```python
from build123d import *

# Parameters (mm, degrees)
SKETCH2_R           = 12.45
BOSS_EXTRUDE1_DEPTH = 16.915
SKETCH6_R           = 11
CUT_EXTRUDE2_DEPTH  = 15.5
BOSS_EXTRUDE2_START = 9
BOSS_EXTRUDE2_DEPTH = 9
SKETCH5_R           = 2.265
CUT_EXTRUDE1_DEPTH  = 33.574986186
CHAMFER1_SIZE       = 0.5
CHAMFER2_SIZE       = 0.5


with BuildPart() as part:
    # Sketch2 → Boss-Extrude1 (new body)
    with BuildSketch(Plane(origin=(0, 0, 0), x_dir=(1, 0, 0), z_dir=(0, 1, 0))):
        with Locations(Location((0, 0, 0), (0, 0, 270))):
            Circle(SKETCH2_R)
    extrude(amount=BOSS_EXTRUDE1_DEPTH)

    # Sketch6 → Cut-Extrude2 (cut)
    with BuildSketch(Plane.XZ):
        with Locations(Location((0, 0, 0), (0, 0, 270))):
            Circle(SKETCH6_R)
    extrude(amount=-CUT_EXTRUDE2_DEPTH, mode=Mode.SUBTRACT)

    # Sketch7 → Boss-Extrude2 (add)
    with BuildSketch(Plane.XZ.offset(-15.5).offset(BOSS_EXTRUDE2_START)):
        with BuildLine():
            Line((-4, 10.246950766), (-4, -10.246950766))
            ThreePointArc((-4, -10.246950766), (-11, 0), (-4, 10.246950766))
        make_face()
        with BuildLine():
            Line((4, 10.246950766), (4, -10.246950766))
            ThreePointArc((4, -10.246950766), (11, 0), (4, 10.246950766))
        make_face()
    extrude(amount=-BOSS_EXTRUDE2_DEPTH)

    # Sketch5 → Cut-Extrude1 (cut, through all)
    with BuildSketch(Plane(origin=(12.45, 0, 0), x_dir=(0, 0, -1), z_dir=(1, 0, 0))):
        with Locations((0, 9.95)):
            Circle(SKETCH5_R)
    extrude(amount=-CUT_EXTRUDE1_DEPTH, mode=Mode.SUBTRACT)

    # Chamfer1
    chamfer1_edges = [part.edges().sort_by_distance(p)[0] for p in [
        (0, 16.915, -12.45),
    ]]
    chamfer(chamfer1_edges, length=CHAMFER1_SIZE)

    # Chamfer2
    chamfer2_edges = [part.edges().sort_by_distance(p)[0] for p in [
        (0, 0, -12.45),
    ]]
    chamfer(chamfer2_edges, length=CHAMFER2_SIZE)


solid = part.part
```
The listing builds one solid part. Answer for the finished solid, in the listing's coordinates (mm). A direction names the side the tool comes from. Coordinates: 2 decimals unless noted, no trailing zeros. Write each loop counter-clockwise with the first axis right and the second up, starting at its lowest first coordinate (ties: lowest second). Pieces come first, ordered by that corner, then holes. Notation, with made-up numbers: (45.25, -11.75) - (57.25, -11.75) arc R32 cw to (57.25, 17.25) - close; hole circle Ø9 at (-10.5, 4). An arc over 180 degrees is marked (long way). Return JSON: item names as keys, results as strings. Group by question number.
1. Which of the six approach directions +Z, -Z, +X, -X, +Y, -Y give full straight-line access (tool end or side, diameter ignored) to faces 1 (the flat face through (7, 6.5, 0)), 2 (the cylindrical face through (-12.154, 8.346, -2.699))?
2. Straight lines are drawn through the part: L1, parallel to X at y = 15.25, z = 3.5; L2, parallel to Y at x = -7.75, z = 0 (3 decimals); L3, parallel to Y at x = -0.25, z = 8.25 (3 decimals). For each, find the intervals that lie inside material, in ascending order.
3. Given pin 1 (2.5 mm diameter, centred on x = 0, z = -4.5, fed in from -Y); pin 2 (7.5 mm diameter, centred on x = -6.5, z = 3, fed in from -Y); pin 3 (4 mm diameter, centred on y = 4, z = -2.5, fed in from +X), each flat-ended and moving along its own axis, determine where each tip first touches the part or whether it passes through.
4. A cutting plane is placed at D-D, the plane x = 0. Determine the outline of the cut face in (y, z) (3 decimals).
5. A cutting plane is placed at A-A, the plane z = 0. Determine the outline of the cut face in (x, y) (3 decimals), plus the area to 3 significant figures.
6. A cutting plane is placed at C-C, the plane y = 13. Determine the outline of the cut face in (x, z), plus the area to 3 significant figures.
7. A cutting plane is placed at B-B, the plane y = 9.95. Determine the outline of the cut face in (x, z) (3 decimals), plus the area to 3 significant figures.
8. Determine the mould class of faces 3 (the flat face through (0, 16.915, 0)), 4 (the flat face through (4, 13, 0)), 5 (the cylindrical face through (8.28, 7.74, 0.49)), 6 (the cylindrical face through (-8.17, 7.74, 0.49)) for opening direction Y: released by +Y, released by -Y, zero draft, split by the parting line, or undercut.
Ans:
{
 "1": {"face 1": "-Y", "face 2": "+Y, -Y"},
 "2": {"L1": "-11.95 to -4, 4 to 11.95", "L2": "6.5 to 7.685, 12.215 to 16.915", "L3": "15.5 to 16.915"},
 "3": {"pin 1": "y = 15.5", "pin 2": "y = 6.5", "pin 3": "x = 12.44"},
 "4": {"outline": "(0, -11.95) - (0.5, -12.45) - (16.415, -12.45) - (16.915, -11.95) - (16.915, 11.95) - (16.415, 12.45) - (0.5, 12.45) - (0, 11.95) - (0, 11) - (15.5, 11) - (15.5, -11) - (0, -11) - close"},
 "5": {"outline": "(-12.45, 0.5) - (-11.95, 0) - (-11, 0) - (-11, 6.5) - (-4, 6.5) - (-4, 7.685) - (-12.45, 7.685) - close; (-12.45, 12.215) - (-4, 12.215) - (-4, 15.5) - (4, 15.5) - (4, 12.215) - (12.45, 12.215) - (12.45, 16.415) - (11.95, 16.915) - (-11.95, 16.915) - (-12.45, 16.415) - close; (4, 6.5) - (11, 6.5) - (11, 0) - (11.95, 0) - (12.45, 0.5) - (12.45, 7.685) - (4, 7.685) - close", "area": "129 mm²"},
 "6": {"outline": "circle Ø24.9 at (0, 0); hole (-4, -10.25) arc R11 ccw to (4, -10.25) - (4, 10.25) arc R11 ccw to (-4, 10.25) - close", "area": "315 mm²"},
 "7": {"outline": "(-12.242, -2.265) arc R12.45 ccw to (12.242, -2.265) - (4, -2.265) - (4, -10.247) arc R11 cw to (-4, -10.247) - (-4, -2.265) - close; (-12.242, 2.265) - (-4, 2.265) - (-4, 10.247) arc R11 cw to (4, 10.247) - (4, 2.265) - (12.242, 2.265) arc R12.45 ccw to start", "area": "239 mm²"},
 "8": {"face 3": "released by +Y", "face 4": "zero draft", "face 5": "undercut", "face 6": "undercut"}
}
